The listing builds one solid part. Answer for the finished solid, in the listing's coordinates (mm). Face numbers are marked on the shaded views. Give positions to 0.01 mm unless a question says otherwise; leave off trailing zeros. Write each loop counter-clockwise with the first axis right and the second up, starting at its lowest first coordinate (ties: lowest second). Pieces come first, ordered by that corner, then holes. Notation, with made-up numbers: (59.5, 57) - (64.5, 57) arc R8 ccw to (64.5, 65) - close; hole circle Ø8 at (73, 24.25). An arc over 180 degrees is marked (long way). One line per item, written item: value. Start each with the question number.
from build123d import *

# Parameters (mm, degrees)
ESQUISSE1_R             = 15
BOSS_EXTRU_1_DEPTH      = 5
ESQUISSE2_R             = 6
BOSS_EXTRU_2_DEPTH      = 1.5
ESQUISSE3_R             = 1.6
ENL_V_MAT_EXTRU_1_DEPTH = 23.186707732
ESQUISSE4_R             = 3.7
ENL_V_MAT_EXTRU_2_DEPTH = 5.5
D_GAGEMENT_M2_51_D      = 2.7


with BuildPart() as part:
    # Esquisse1 → Boss.-Extru.1 (new body)
    with BuildSketch(Plane(origin=(0, 0, 0), x_dir=(1, 0, 0), z_dir=(0, 1, 0))):
        with Locations(Location((0, 0, 0), (0, 0, 270))):
            Circle(ESQUISSE1_R)
    extrude(amount=BOSS_EXTRU_1_DEPTH)

    # Esquisse2 → Boss.-Extru.2 (add)
    with BuildSketch(Plane(origin=(0, 5, 0), x_dir=(1, 0, 0), z_dir=(0, 1, 0))):
        with Locations(Location((0, 0, 0), (0, 0, 270))):
            Circle(ESQUISSE2_R)
    extrude(amount=BOSS_EXTRU_2_DEPTH)

    # Esquisse3 → Enlèv. mat.-Extru.1 (cut, through all)
    with BuildSketch(Plane.XZ):
        with Locations(Location((0, 0, 0), (0, 0, 270))):
            Circle(ESQUISSE3_R)
    extrude(amount=-ENL_V_MAT_EXTRU_1_DEPTH, mode=Mode.SUBTRACT)

    # Esquisse4 → Enlèv. mat.-Extru.2 (cut)
    with BuildSketch(Plane.XZ):
        with Locations(Location((0, 0, 0), (0, 0, 270))):
            Circle(ESQUISSE4_R)
    extrude(amount=-ENL_V_MAT_EXTRU_2_DEPTH, mode=Mode.SUBTRACT)

    # Dégagement M2.51 (through all)
    with Locations(Plane(origin=(0, 5, 0), x_dir=(1, 0, 0), z_dir=(0, 1, 0))):
        with Locations((0, 0), (-12, 0), (-8.485281374, 8.485281374), (0, 12), (8.485281374, 8.485281374), (12, 0), (8.485281374, -8.485281374), (0, -12), (-8.485281374, -8.485281374)):
            Hole(D_GAGEMENT_M2_51_D / 2)


solid = part.part
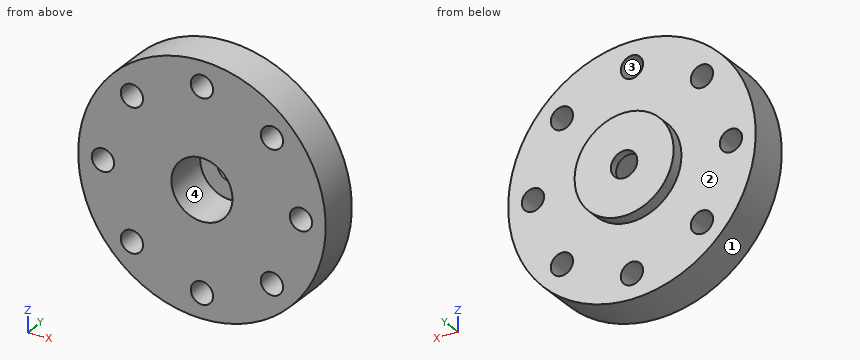
Item 1: Each of these flat-tipped pins is pushed along its axis until it touches: pin 1 Ø3 at (x, y) = (-7.5, 1) entering from +Z; pin 2 Ø1 at (y, z) = (3.5, -9.5) entering from -X. Where does it stop, or does it pass through?
Item 2: Straight lines are drawn through the part: line 1 along Y through (x, z) = (7, -4); line 2 along X through (y, z) = (1.8, -12); line 3 along X through (y, z) = (4.25, 8.5). For each, find the intervals that lie inside material, in ascending order.
Item 3: The mould has two halves that part along Z. Classify the marked faces 1, 2, 3 and 4: +Z half, -Z half, draft (parallel to the pull), parting line (faces both ways), or undercut.
Item 4: Find section B-B on z = 12. Determine the outline of the cut face in (x, y).
Item 5: Find section A-A on x = 12. Determine the outline of the cut face in (y, z).
Item 6: Find section C-C on z = 0. Determine the outline of the cut face in (x, y).
Item 7: Find section D-D on z = -9.25. Determine the outline of the cut face in (x, y).
Values:
1. pin 1: z = 13.75
1. pin 2: x = -12
2. line 1: 0 to 5
2. line 2: -9 to -1.35, 1.35 to 9
2. line 3: -12.36 to -9.84, -7.14 to 7.14, 9.84 to 12.36
3. face 1: parting line
3. face 2: draft
3. face 3: undercut
3. face 4: undercut
4. outline: (-9, 0) - (-1.35, 0) - (-1.35, 5) - (-9, 5) - close; (1.35, 0) - (9, 0) - (9, 5) - (1.35, 5) - close
5. outline: (0, -9) - (5, -9) - (5, -1.35) - (0, -1.35) - close; (0, 1.35) - (5, 1.35) - (5, 9) - (0, 9) - close
6. outline: (-15, 0) - (-13.35, 0) - (-13.35, 5) - (-15, 5) - close; (-10.65, 0) - (-3.7, 0) - (-3.7, 5.5) - (-1.6, 5.5) - (-1.6, 6.5) - (-6, 6.5) - (-6, 5) - (-10.65, 5) - close; (1.6, 5.5) - (3.7, 5.5) - (3.7, 0) - (10.65, 0) - (10.65, 5) - (6, 5) - (6, 6.5) - (1.6, 6.5) - close; (13.35, 0) - (15, 0) - (15, 5) - (13.35, 5) - close
7. outline: (-11.81, 0) - (-9.6, 0) - (-9.6, 5) - (-11.81, 5) - close; (-7.37, 0) - (7.37, 0) - (7.37, 5) - (-7.37, 5) - close; (9.6, 0) - (11.81, 0) - (11.81, 5) - (9.6, 5) - close
